Verification items for the finished model (mm, model axes). A direction names the side the tool comes from. Give positions to 0.01 mm unless a question says otherwise; leave off trailing zeros. Loops run counter-clockwise (first coordinate to the right, second up) from the corner with the lowest first, then second, coordinate; pieces in that order, holes last. Notation, with made-up numbers: (6.5, -19.5) - (50.5, -19.5) arc R17 cw to (50.5, -15.5) - close; hole circle Ø8 at (-8, 58.25). An arc over 180 degrees is marked (long way). One line per item, written item: value. Start each with the question number.
1. Mould release check, pull along X, two halves, no side actions. Record for faces 5 (the flat face through (61, 51, -7)), 6 (the cylindrical face through (11, 42, -7)), 7 (the flat face through (48.025, -1, -7)): pulls with the +X half, pulls with the -X half, needs draft (parallel to the pull), parting line crosses it, or undercut.
2. Gauge pin test, flat ends, axial feed: pin 1 (1.4 mm diameter, centred on x = 121, y = 0, fed in from -Z); pin 2 (6 mm diameter, centred on y = 10, z = -10.5, fed in from +X); pin 3 (6.5 mm diameter, centred on x = 0, y = 0, fed in from -Z); pin 4 (3 mm diameter, centred on x = 0, y = 0, fed in from -Z). Record the tip position at first contact, or that the pin passes through.
3. Sectioned sample at A-A (x = 4.5). Record the cut outline in (y, z).
4. Sectioned sample at C-C (z = -3). Count the separate pieces of the cut face and the enclosed holes in it, plus the area to 3 significant figures.
5. Scan lines: L1, parallel to X at y = 0, z = -3 (3 decimals); L2, parallel to Y at x = 0, z = -13.3; L3, parallel to Y at x = 121, z = -7. Record each from-to range of solid material in increasing order. Write a range as [from, to].
6. Access from +Z, -Z, +X, -X, +Y, -Y to the whole of each face (thin tool, end or side, straight path). Record for faces 1 (the flat face through (64.725, 0, -7)), 2 (the cylindrical face through (24, 36, -7)), 3 (the flat face through (2, 3, -7)), 4 (the flat face through (123, 3, -7)).
7. Sectioned sample at B-B (y = 29). Record the cut outline in (x, z).
8. Sectioned sample at D-D (y = 41). Record the cut outline in (x, z).
from build123d import *

# Parameters (mm, degrees)
EXTRUDE_1_DEPTH               = 15
HOLE_WIZARD_M21_D             = 2.4
HOLE_WIZARD_M21_CSINK_D       = 2.45
HOLE_WIZARD_M21_CSINK_ANGLE   = 90
HOLE_WIZARD_5_0_1_D           = 5
HOLE_WIZARD_5_0_1_DEPTH       = 3.497848452
HOLE_WIZARD_5_0_1_CSINK_D     = 5.05
HOLE_WIZARD_5_0_1_CSINK_ANGLE = 90
HOLE_WIZARD_5_0_1_TIP         = 1.502151548


with BuildPart() as part:
    # Эскиз9 → Бобышка-Вытянуть1 (new body)
    with BuildSketch(Plane.XY):
        with BuildLine():
            Line((-1.706e-06, -5.00000143), (48.02500155, -5.00000143))
            Line((48.02500155, -5.00000143), (48.02500155, 3.9624))
            ThreePointArc((48.02500155, 3.9624), (48.610787988, 5.376613562), (50.02500155, 5.9624))
            Line((50.02500155, 5.9624), (62.72500155, 5.9624))
            ThreePointArc((62.72500155, 5.9624), (64.139215112, 5.376613562), (64.72500155, 3.9624))
            Line((64.72500155, 3.9624), (64.72500155, -5.00000143))
            Line((64.72500155, -5.00000143), (120.99999946, -5.00000143))
            ThreePointArc((120.99999946, -5.00000143), (124.535533366, -3.535535336), (125.99999946, -1.43e-06))
            Line((125.99999946, -1.43e-06), (125.99999946, 2.99999857))
            Line((125.99999946, 2.99999857), (120.09775193, 2.99999857))
            ThreePointArc((120.09775193, 2.99999857), (116.562218024, 4.464464664), (115.09775193, 7.99999857))
            Line((115.09775193, 7.99999857), (115.09775193, 37.99999857))
            ThreePointArc((115.09775193, 37.99999857), (116.562218024, 41.535532476), (120.09775193, 42.99999857))
            Line((120.09775193, 42.99999857), (125.99999946, 42.99999857))
            Line((125.99999946, 42.99999857), (125.99999946, 45.99999857))
            ThreePointArc((125.99999946, 45.99999857), (124.535533366, 49.535532476), (120.99999946, 50.99999857))
            Line((120.99999946, 50.99999857), (-1.706e-06, 50.99999857))
            ThreePointArc((-1.706e-06, 50.99999857), (-3.535534858, 49.535532064), (-5.00000054, 45.99999857))
            Line((-5.00000054, 45.99999857), (-5.00000054, 42.99999857))
            Line((-5.00000054, 42.99999857), (7.999998294, 42.99999857))
            ThreePointArc((7.999998294, 42.99999857), (11.5355322, 41.535532476), (12.999998294, 37.99999857))
            Line((12.999998294, 37.99999857), (12.999998294, 7.99999857))
            ThreePointArc((12.999998294, 7.99999857), (11.5355322, 4.464464664), (7.999998294, 2.99999857))
            Line((7.999998294, 2.99999857), (-5.000001706, 2.99999857))
            Line((-5.000001706, 2.99999857), (-5.000001706, -1.43e-06))
            ThreePointArc((-5.000001706, -1.43e-06), (-3.535535612, -3.535535336), (-1.706e-06, -5.00000143))
        make_face()
        with BuildLine():
            Line((27.999998294, 37.99999857), (100.09775193, 37.99999857))
            ThreePointArc((100.09775193, 37.99999857), (103.633285836, 36.535532476), (105.09775193, 32.99999857))
            Line((105.09775193, 32.99999857), (105.09775193, 12.99999857))
            ThreePointArc((105.09775193, 12.99999857), (103.633285836, 9.464464664), (100.09775193, 7.99999857))
            Line((100.09775193, 7.99999857), (27.999998294, 7.99999857))
            ThreePointArc((27.999998294, 7.99999857), (24.464464388, 9.464464664), (22.999998294, 12.99999857))
            Line((22.999998294, 12.99999857), (22.999998294, 32.99999857))
            ThreePointArc((22.999998294, 32.99999857), (24.464464388, 36.535532476), (27.999998294, 37.99999857))
        make_face(mode=Mode.SUBTRACT)
    extrude(amount=-EXTRUDE_1_DEPTH)

    # Отверстие с зазором M21 (through all)
    with Locations(Plane.XY):
        with Locations((1.27e-06, 45.99999944), (0, 0), (120.9999993, -1.27e-06), (120.9999993, 45.99999944)):
            CounterSinkHole(HOLE_WIZARD_M21_D / 2, HOLE_WIZARD_M21_CSINK_D / 2, counter_sink_angle=HOLE_WIZARD_M21_CSINK_ANGLE)

    # Отверстия под штифты Ø5.0 мм1
    with Locations(Plane(origin=(0, 0, -15), x_dir=(-1, 0, 0), z_dir=(0, 0, -1))):
        with Locations((-120.9999993, -1.27e-06), (-120.9999993, 45.99999944), (-1.27e-06, 45.99999944), (0, 0), (-55.116594528, 0)):
            CounterSinkHole(HOLE_WIZARD_5_0_1_D / 2, HOLE_WIZARD_5_0_1_CSINK_D / 2, depth=HOLE_WIZARD_5_0_1_DEPTH, counter_sink_angle=HOLE_WIZARD_5_0_1_CSINK_ANGLE)
            with Locations((0, 0, -(HOLE_WIZARD_5_0_1_DEPTH + HOLE_WIZARD_5_0_1_TIP / 2))):  # 118° drill point
                Cone(0, HOLE_WIZARD_5_0_1_D / 2, HOLE_WIZARD_5_0_1_TIP, mode=Mode.SUBTRACT)


solid = part.part
Results are:
1. face 5: needs draft
1. face 6: pulls with the -X half
1. face 7: undercut
2. pin 1: passes through
2. pin 2: stops at x = 115.2
2. pin 3: stops at z = -15
2. pin 4: stops at z = -10.9
3. outline: (-5, -15) - (3, -15) - (3, 0) - (-5, 0) - close; (43, -15) - (51, -15) - (51, 0) - (43, 0) - close
4. separate pieces: 1
4. enclosed holes: 5
4. area: 3,540 mm^2
5. L1: x = [-5, -1.2], [1.2, 48.025], [64.725, 119.8], [122.2, 126]
5. L2: y = [-5, -2.5], [2.5, 3], [43, 43.5], [48.5, 51]
5. L3: y = [-5, -1.2], [1.2, 3], [43, 44.8], [47.2, 51]
6. face 1: +Z, -Z, -Y
6. face 2: +Z, -Z
6. face 3: +Z, -Z, -X
6. face 4: +Z, -Z, +X
7. outline: (13, -15) - (23, -15) - (23, 0) - (13, 0) - close; (105.1, -15) - (115.1, -15) - (115.1, 0) - (105.1, 0) - close
8. outline: (12, -15) - (116.1, -15) - (116.1, 0) - (12, 0) - close
